Job drawing, mm, ordinate dimensions from the low corner. One solid piece. Coordinates: 2 decimals unless noted, no trailing zeros. Order: outer loops, then holes, each group sorted by start corner. A loop starts at its lowest first (then second) coordinate and runs counter-clockwise, first axis right, second up. Notation, with made-up numbers: (46.25, 36.25) - (54.25, 36.25) arc R12 ccw to (54.25, 46.25) - close; hole circle Ø9 at (14.5, 71.5). An arc over 180 degrees is marked (long way). Return JSON: item names as keys, results as strings.
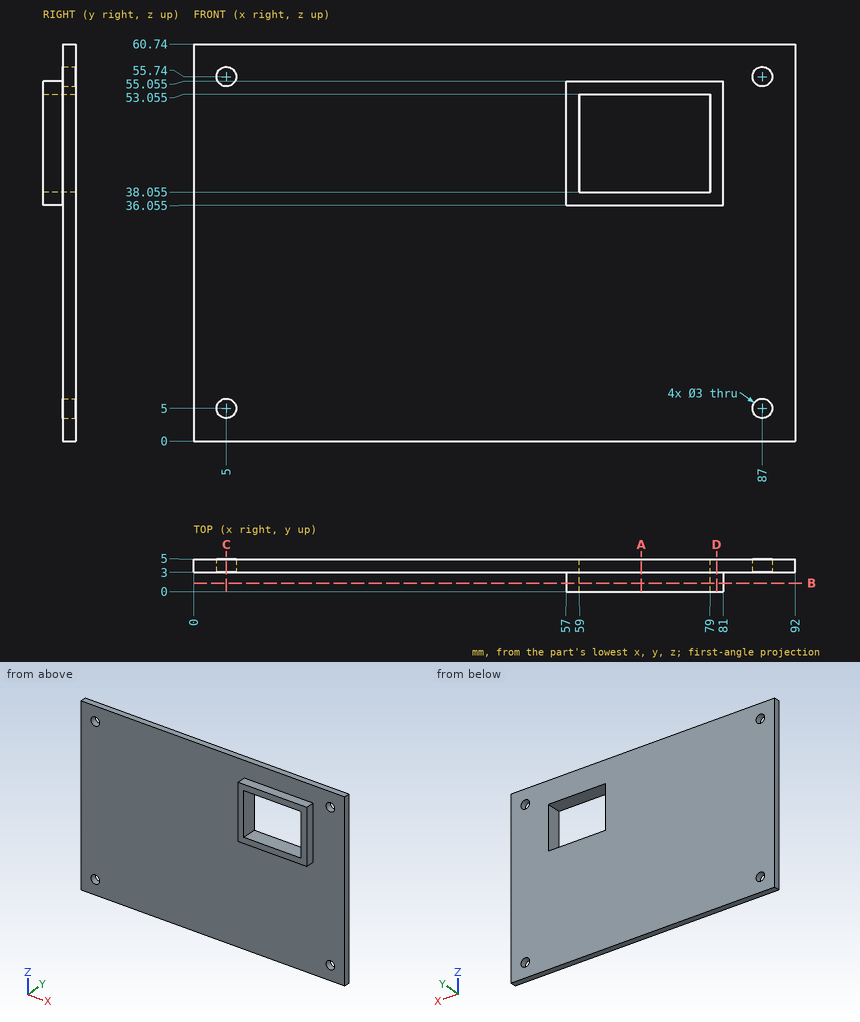
1. Drop flat-ended pins along their axis: pin 1 (1.8 mm diameter, centred on x = 5, z = 55.74, fed in from +Y); pin 2 (1.5 mm diameter, centred on y = 1, z = 49, fed in from -X); pin 3 (1.5 mm diameter, centred on x = 63.5, y = 1, fed in from -Z) (3 decimals); pin 4 (6 mm diameter, centred on x = 25.5, z = 46.5, fed in from -Y). Give the stop position or say it passes through.
Check values:
{"pin 1": "through", "pin 2": "x = 57", "pin 3": "z = 36.055", "pin 4": "y = 3"}
2. Cut at A-A on x = 68.5. Give the cut face in (y, z) (3 decimals).
Check values:
{"outline": "(0, 36.055) - (3, 36.055) - (3, 0) - (5, 0) - (5, 38.055) - (0, 38.055) - close; (0, 53.055) - (5, 53.055) - (5, 60.74) - (3, 60.74) - (3, 55.055) - (0, 55.055) - close"}
3. Cut at C-C on x = 5. Give the cut face in (y, z), plus the area to 3 significant figures.
Check values:
{"outline": "(3, 0) - (5, 0) - (5, 3.5) - (3, 3.5) - close; (3, 6.5) - (5, 6.5) - (5, 54.24) - (3, 54.24) - close; (3, 57.24) - (5, 57.24) - (5, 60.74) - (3, 60.74) - close", "area": "109 mm²"}
4. Cut at B-B on y = 1.3. Give the cut face in (x, z) (3 decimals), plus the area to 3 significant figures.
Check values:
{"outline": "(57, 36.055) - (81, 36.055) - (81, 55.055) - (57, 55.055) - close; hole (59, 38.055) - (79, 38.055) - (79, 53.055) - (59, 53.055) - close", "area": "156 mm²"}
5. Probe L1, parallel to Z at x = 5, y = 3.65; L2, parallel to X at y = 4.15, z = 5; L3, parallel to X at y = 3.5, z = 49.5. List the from-to ranges inside material, lowest first.
Check values:
{"L1": "0 to 3.5, 6.5 to 54.24, 57.24 to 60.74", "L2": "0 to 3.5, 6.5 to 85.5, 88.5 to 92", "L3": "0 to 59, 79 to 92"}
6. Cut at D-D on x = 80. Give the cut face in (y, z) (3 decimals).
Check values:
{"outline": "(0, 36.055) - (3, 36.055) - (3, 0) - (5, 0) - (5, 60.74) - (3, 60.74) - (3, 55.055) - (0, 55.055) - close"}
